Input: part model. Units: mm. Frame: model coordinates. Face numbers are marked on the shaded views. A direction names the side the tool comes from. Coordinates: 2 decimals unless noted, no trailing zeros. Write each loop counter-clockwise with the first axis right and the second up, starting at its lowest first coordinate (ties: lowest second). Pieces come first, ordered by that corner, then holes. Notation, with made-up numbers: (-0.5, 10) - (38.5, 10) arc R11 ccw to (38.5, 14) - close; hole circle Ø2 at (51.5, 65.5). An arc over 180 degrees is marked (long way). One line per question, with ' | ' between items. Start each with the question number.
1) Section query B-B on x = 0. Return loops of the section in (y, z).
2) Section query C-C on z = -5.5. Return loops of the section in (x, y).
3) Line query: line 1 (Y direction, x = 0, z = -5.75); line 2 (Y direction, x = 6.5, z = -10.25); line 3 (X direction, y = -8.5, z = -7.75). Output: solid intervals per line, ascending.
4) Reachability of the marked faces 5 and 6 from +Z, -Z, +X, -X, +Y, -Y: full face, straight path, thin tool, end or side. Return the list, or none.
5) Draft query along Y for the marked faces 1, 2, 3 and 4. Return one class per face: released by +Y, released by -Y, zero draft, split by the parting line, or undercut.
6) Section query D-D on y = 12. Return loops of the section in (x, z).
7) Section query A-A on y = -2. Return loops of the section in (x, z).
8) First-contact query: P1, Ø1.5, axis at y = -10, z = -5.5, coming from the -X side; P2, Ø1.5, axis at y = -8.5, z = -11, coming from the -X side; P3, Ø3, axis at x = 12.5, z = -11, coming from the -Y side. Flat tips, straight axial feed; report the tip coordinate or a pass-through.
Autodesk Inventor part; units mm, degrees
ref_plane "YZ Plane" through (0, 0, 0) normal (1, 0, 0) x (0, 1, 0)
ref_plane "XZ Plane" through (0, 0, 0) normal (0, 1, 0) x (-1, 0, 0)
ref_plane "XY Plane" through (0, 0, 0) normal (0, 0, 1) x (1, 0, 0)
ref_plane "Work Plane4" through (21.2718, 3.7508, -2.4) normal (0, 0, -1) x (-1, 0, 0)
sketch "Sketch5" plane through (21.2718, 3.7508, -2.4) normal (0, 0, -1) x (-1, 0, 0)
  arc A0 (24.639, -2.4773) -> (21.9352, 21.2492) centre (13.3117, 8.2492) ccw
  arc A1 (23.0748, -0.6348) -> (20.6085, 19.2492) centre (13.3118, 8.2492) ccw
  arc A2 (23.0687, -6.8701) -> (24.639, -2.4773) centre (21.2719, -3.7507) ccw
  arc A3 (23.0687, -6.8701) -> (41.5221, -14.6763) centre (35.6441, -2.8572) ccw
  line L0 (41.5221, -14.6763) -> (42.5908, -16.8253)
  arc A4 (20.691, -7.3035) -> (42.5908, -16.8253) centre (35.6441, -2.8572) ccw
  arc A5 (17.672, -3.7474) -> (20.691, -7.3035) centre (21.2719, -3.7507) ccw
  arc A6 (18.4854, -1.4715) -> (-0.7105, -15.6763) centre (14.8594, -16.6442) ccw
  arc A7 (23.0748, -0.6348) -> (18.4854, -1.4715) centre (21.2719, -3.7507) ccw
  arc A8 (17.672, -3.7474) -> (1.6849, -15.8253) centre (14.8595, -16.6443) ccw
  line L1 (1.6849, -15.8253) -> (-0.7105, -15.6763)
  line L2 (20.6085, 19.2492) -> (21.9352, 21.2492)
  point P0 (21.2718, -3.7508)
  dimension "d11" = 3.5999
  dimension "d13" = 13.2001
  dimension "d14" = 15.6002
  dimension "d15" = 13.2
  dimension "d16" = 15.5999
  dimension "d17" = 13.2001
  dimension "d18" = 15.6001
extrude "Extrusion2" add sketch "Sketch5" along normal blind 14
sketch "Sketch6" plane through (21.2718, 3.7508, -2.4) normal (0, 0, 1) x (1, 0, 0)
  circle A0 centre (-21.2718, -3.7508) radius 1.5
  dimension "d21" = 3
hole "Hole1" at (0, 0, -2.4) direction (0, 0, -1) diameter 1 depth 14 tip angle 118
properties part number "pump_impeller_rev_2"
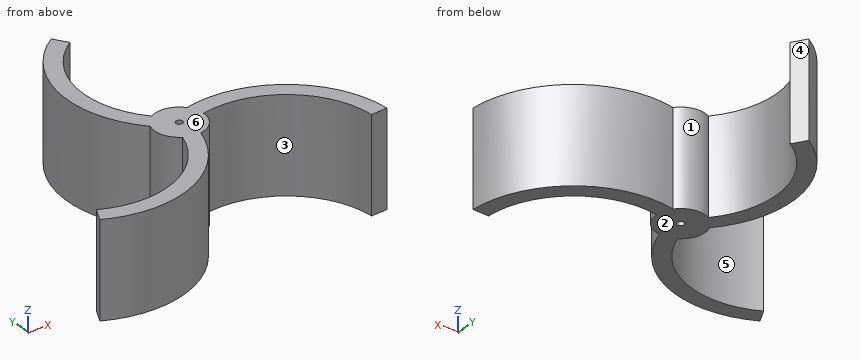
Answer key:
1) outline: (-5.17, -16.4) - (-0.5, -16.4) - (-0.5, -2.4) - (-5.17, -2.4) - close; (0.5, -16.4) - (3.6, -16.4) - (3.6, -2.4) - (0.5, -2.4) - close; (22.53, -16.4) - (24, -16.4) - (24, -2.4) - (22.53, -2.4) - close
2) outline: (-21.32, -13.07) arc R15.6 ccw to (0.58, -3.55) arc R3.6 ccw to (3.6, 0) arc R13.2 cw to (19.59, -12.07) - (21.98, -11.93) arc R15.6 ccw to (2.79, 2.28) arc R3.6 ccw to (-1.8, 3.12) arc R13.2 cw to (0.66, 23) - (-0.66, 25) arc R15.6 ccw to (-3.37, 1.27) arc R3.6 ccw to (-1.8, -3.12) arc R13.2 cw to (-20.25, -10.93) - close; hole circle Ø1 at (0, 0)
3) line 1: -5.17 to -0.5, 0.5 to 3.6, 22.53 to 24 | line 2: 0.31 to 2.71 | line 3: -5.1 to -1.92, 18.86 to 21.38
4) face 5: +Z, -Z | face 6: +Z, +X, -X, +Y, -Y
5) face 1: undercut | face 2: zero draft | face 3: released by -Y | face 4: released by +Y
6) outline: (-7.64, -16.4) - (-5.24, -16.4) - (-5.24, -2.4) - (-7.64, -2.4) - close
7) outline: (-2.99, -16.4) - (2.99, -16.4) - (2.99, -2.4) - (-2.99, -2.4) - close; (13.87, -16.4) - (17.58, -16.4) - (17.58, -2.4) - (13.87, -2.4) - close
8) P1: x = -8.15 | P2: x = -5.93 | P3: y = -2.09
